The figure shows three views and two pictorial views of one solid part (mm, origin at its lowest corner). Answer the questions. Give positions to 0.01 mm unless a question says otherwise; leave off trailing zeros. Loops run counter-clockwise (first coordinate to the right, second up) from the corner with the lowest first, then second, coordinate; pieces in that order, holes last. Notation, with made-up numbers: (-33.75, 20.5) - (-15.75, 20.5) arc R18 ccw to (-15.75, 32.5) - close; hole circle Ø1 at (56.25, 33.5). An arc over 180 degrees is marked (long way). One line per question, with ' | ' between items.
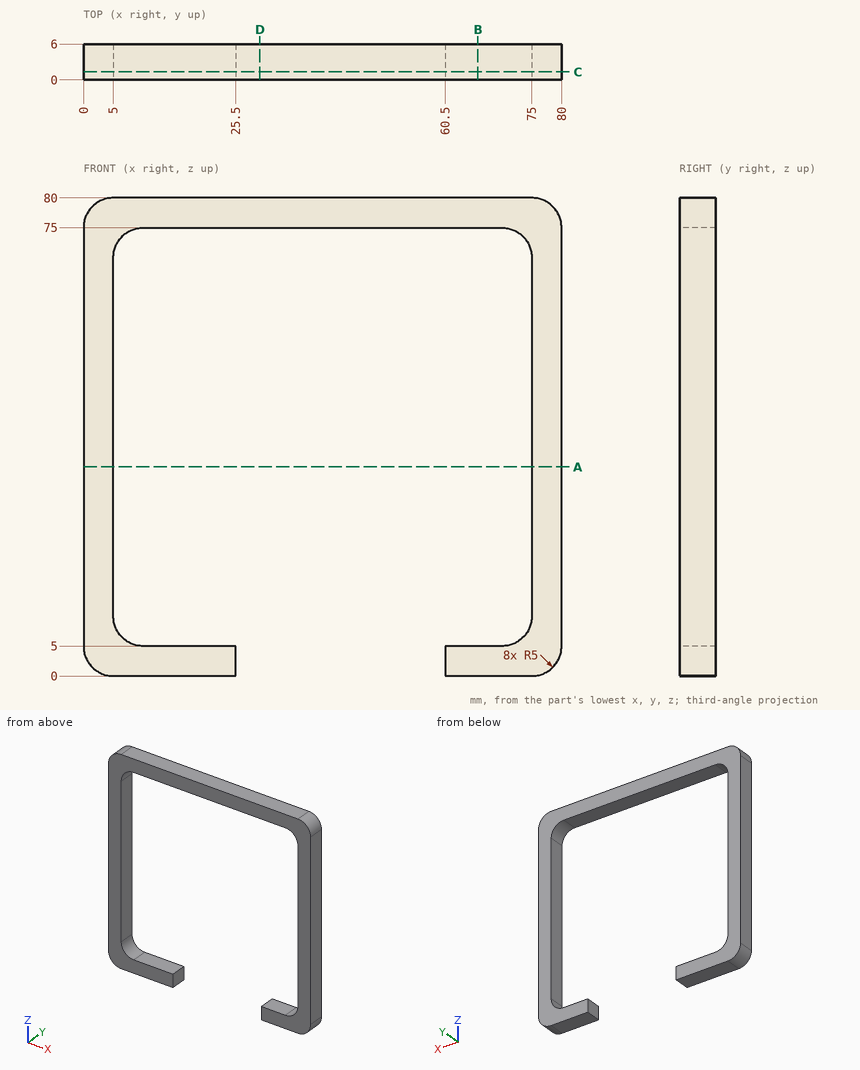
1. Find section D-D on x = 29.5. Write down the section's boundary in (y, z).
Evaluation:
outline: (0, 75) - (6, 75) - (6, 80) - (0, 80) - close
2. Find section B-B on x = 66. Write down the section's boundary in (y, z), then the cut area to 3 significant figures.
Evaluation:
outline: (0, 0) - (6, 0) - (6, 5) - (0, 5) - close; (0, 75) - (6, 75) - (6, 80) - (0, 80) - close | area: 60.0 mm2
3. Find section A-A on z = 35. Write down the section's boundary in (x, y), then the cut area to 3 significant figures.
Evaluation:
outline: (0, 0) - (5, 0) - (5, 6) - (0, 6) - close; (75, 0) - (80, 0) - (80, 6) - (75, 6) - close | area: 60.0 mm2
4. A flat-ended cylindrical pin translates along its axis: pin 1 (1.5 mm diameter, centred on y = 2.5, z = 3.5, fed in from -X). Find the tip coordinate at first contact, or state that the pin passes through.
Evaluation:
pin 1: x = 0.06
5. Consider L1, parallel to X at y = 0.8, z = 50; L2, parallel to Z at x = 35, y = 4.9. Determine where each line is inside the solid, lowest interval first.
Evaluation:
L1: 0 to 5, 75 to 80 | L2: 75 to 80
6. Find section C-C on y = 1.35. Write down the section's boundary in (x, z).
Evaluation:
outline: (0, 5) arc R5 ccw to (5, 0) - (25.5, 0) - (25.5, 5) - (10, 5) arc R5 cw to (5, 10) - (5, 70) arc R5 cw to (10, 75) - (70, 75) arc R5 cw to (75, 70) - (75, 10) arc R5 cw to (70, 5) - (60.5, 5) - (60.5, 0) - (75, 0) arc R5 ccw to (80, 5) - (80, 75) arc R5 ccw to (75, 80) - (5, 80) arc R5 ccw to (0, 75) - close
